Verification items for the finished model (mm, model axes). A direction names the side the tool comes from. Coordinates: 2 decimals unless noted, no trailing zeros. Order: outer loops, then holes, each group sorted by start corner. A loop starts at its lowest first (then second) coordinate and runs counter-clockwise, first axis right, second up. Notation, with made-up numbers: M 82,67.25 L 124,67.25 A17 ccw 124,78.25 Z; hole C 66,-33.75 d8. An arc over 180 degrees is marked long. Answer as a JSON object with one key per item and string values. Group by question number.
(1) Cross-section at C-C (y = -20). Enter the section's corners in (x, z).
(2) Gauge pin test, flat ends, axial feed: pin 1 Ø2.5 at (y, z) = (-31.5, 1.5) entering from +X; pin 2 Ø2.5 at (x, z) = (-23.5, 1.5) entering from +Y; pin 3 Ø2.5 at (x, z) = (-49, 2.5) entering from -Y. Record the tip position at first contact, or that the pin passes through.
(3) Access from +Z, -Z, +X, -X, +Y, -Y to the whole of each face (thin tool, end or side, straight path). Record for faces 1 (the face through (50, 25, 2)), 2 (the face through (-12.5, 32, 2)), 3 (the face through (45, -18, 2)).
(4) Cross-section at B-B (x = 17). Enter the section's corners in (y, z).
(5) Material ranges on line 1 (X direction, y = -32, z = 2.05); line 2 (Y direction, x = -50, z = 3.7); line 3 (X direction, y = 17, z = 2.4), recorded low to high.
(6) Mould release check, pull along Y, two halves, no side actions. Record for faces 4 (the face through (-20, 30, 2)), 5 (the face through (50, 10, 2)), 6 (the face through (12.5, -33, 2)): released by +Y, released by -Y, zero draft, split by the parting line, or undercut.
from build123d import *

# Parameters (mm, degrees)
ESQUISSE1_W             = 110
ESQUISSE1_H             = 70
BOSS_EXTRU_1_DEPTH      = 5
ESQUISSE6_W             = 10
ESQUISSE6_H             = 35
ESQUISSE6_H_2           = 15
ESQUISSE6_W_2           = 15
ESQUISSE6_H_3           = 5
ENL_V_MAT_EXTRU_2_DEPTH = 5


with BuildPart() as part:
    # Esquisse1 → Boss.-Extru.1 (new body)
    with BuildSketch(Plane.XY):
        Rectangle(ESQUISSE1_W, ESQUISSE1_H)
    extrude(amount=BOSS_EXTRU_1_DEPTH)

    # Esquisse6 → Enlèv. mat.-Extru.2 (cut)
    with BuildSketch(Plane(origin=(0, 0, 0), x_dir=(-1, 0, 0), z_dir=(0, 0, -1))):
        with Locations((-50, -17.5)):
            Rectangle(ESQUISSE6_W, ESQUISSE6_H)
        with Locations((50, -17.5)):
            Rectangle(ESQUISSE6_W, ESQUISSE6_H)
        with Locations((-50, 17.5)):
            Rectangle(ESQUISSE6_W, ESQUISSE6_H_2)
        with Locations((50, 17.5)):
            Rectangle(ESQUISSE6_W, ESQUISSE6_H_2)
        with Locations((-20, 32.5)):
            Rectangle(ESQUISSE6_W_2, ESQUISSE6_H_3)
        with Locations((20, 32.5)):
            Rectangle(ESQUISSE6_W_2, ESQUISSE6_H_3)
        with Locations((-20, -32.5)):
            Rectangle(ESQUISSE6_W_2, ESQUISSE6_H_3)
        with Locations((20, -32.5)):
            Rectangle(ESQUISSE6_W_2, ESQUISSE6_H_3)
    extrude(amount=-ENL_V_MAT_EXTRU_2_DEPTH, mode=Mode.SUBTRACT)


solid = part.part
Taken from the geometry:
{
 "1": {"outline": "M -45,0 L 45,0 L 45,5 L -45,5 Z"},
 "2": {"pin 1": "stops at x = 45", "pin 2": "stops at y = 30", "pin 3": "stops at y = 0"},
 "3": {"face 1": "+Z, -Z, +X", "face 2": "+Z, -Z, +Y", "face 3": "+Z, -Z, +X, -Y"},
 "4": {"outline": "M -30,0 L 30,0 L 30,5 L -30,5 Z"},
 "5": {"line 1": "x = -45 to -27.5, -12.5 to 12.5, 27.5 to 45", "line 2": "y = 0 to 10, 25 to 35", "line 3": "x = -45 to 45"},
 "6": {"face 4": "released by +Y", "face 5": "undercut", "face 6": "zero draft"}
}
